from build123d import *

# Parameters (mm, degrees)
BOSS_EXTRUDE1_DEPTH          = 381
F_10_0_1935_DIAMETER_HOLE2_D = 4.9149
F_10_0_1935_DIAMETER_HOLE4_D = 4.9149


with BuildPart() as part:
    # Sketch2 → Boss-Extrude1 (new body)
    with BuildSketch(Plane.XY):
        Polygon((0, 0), (0, 31.75), (1.5875, 31.75), (1.5875, 1.5875), (31.75, 1.5875), (31.75, 0), align=None)
    extrude(amount=BOSS_EXTRUDE1_DEPTH)

    # #10 (0.1935) Diameter Hole2 (through all)
    with Locations(Plane.ZY):
        with Locations((355.6, 15.875), (25.4, 15.875), (190.5, 15.875)):
            Hole(F_10_0_1935_DIAMETER_HOLE2_D / 2)

    # #10 (0.1935) Diameter Hole4 (through all)
    with Locations(Plane(origin=(0, 0, 0), x_dir=(-1, 0, 0), z_dir=(0, -1, 0))):
        with Locations((-15.875, -366.395), (-15.875, -190.5), (-15.875, -25.4), (-15.875, -355.6), (-15.875, -14.605)):
            Hole(F_10_0_1935_DIAMETER_HOLE4_D / 2)


solid = part.part
Work out the finished part from the listing and answer in its coordinate system (mm). A direction names the side the tool comes from. Give positions to 0.01 mm unless a question says otherwise; leave off trailing zeros. Order: outer loops, then holes, each group sorted by start corner. A loop starts at its lowest first (then second) coordinate and runs counter-clockwise, first axis right, second up. Notation, with made-up numbers: (-29.75, 63.5) -> (-1.75, 63.5) arc R9 cw to (-1.75, 73.5) -> close; hole circle Ø6 at (-14, 84). An arc over 180 degrees is marked (long way). Answer as a JSON object with one key per item and string values. Group by question number.
1. A tool of negligible diameter and unlimited length cuts with its end or side. For faces 1 (the flat face through (16.1, 0, 187.8)), 2 (the flat face through (16.5, 1.588, 187.8)), from which of +Z, -Z, +X, -X, +Y, -Y can it reach the whole face along a straight path? Write none if from no direction.
2. Flat-ended cylindrical pins translate along their axes: pin 1 Ø2 at (y, z) = (18.5, 178) entering from +X; pin 2 Ø3 at (x, y) = (14, 4) entering from +Z; pin 3 Ø5.5 at (x, z) = (15.875, 25.4) entering from +Y. Find the tip coordinate at first contact, or state that the pin passes through.
3. Section B-B on x = 7.5 is taken. Determine the outline of the cut face in (y, z), plus the area to 3 significant figures.
4. Consider line 1 along Y through (x, z) = (1.05, 25.4); line 2 along Y through (x, z) = (23.5, 219). Determine where each line is inside the solid, lowest interval first. Write a range as [from, to].
5. Section A-A on z = 310 is taken. Determine the outline of the cut face in (x, y), plus the area to 3 significant figures.
Result sheet:
{
 "1": {"face 1": "+Z, -Z, +X, -X, -Y", "face 2": "+Z, -Z, +X, +Y"},
 "2": {"pin 1": "stops at x = 1.59", "pin 2": "passes through", "pin 3": "stops at y = 1.59"},
 "3": {"outline": "(0, 0) -> (1.59, 0) -> (1.59, 381) -> (0, 381) -> close", "area": "605 mm^2"},
 "4": {"line 1": "y = [0, 13.42], [18.33, 31.75]", "line 2": "y = [0, 1.59]"},
 "5": {"outline": "(0, 0) -> (31.75, 0) -> (31.75, 1.59) -> (1.59, 1.59) -> (1.59, 31.75) -> (0, 31.75) -> close", "area": "98.3 mm^2"}
}
